The model under review builds one solid part; all positions refer to its coordinate system, in mm. A direction names the side the tool comes from. Coordinates: 2 decimals unless noted, no trailing zeros. Loops run counter-clockwise (first coordinate to the right, second up) from the corner with the lowest first, then second, coordinate; pieces in that order, holes last. Notation, with made-up numbers: M 82.5,32 L 90.5,32 A33 cw 90.5,62 Z; hole C 69.25,37 d9. An arc over 180 degrees is marked long. One line per item, written item: value.
```python
from build123d import *

# Parameters (mm, degrees)
SKETCH1_R           = 12.5
SKETCH1_R_2         = 9
BOSS_EXTRUDE1_DEPTH = 27.5
SKETCH1_3_R         = 9
BOSS_EXTRUDE2_DEPTH = 266.1
SKETCH2_R           = 12.5
BOSS_EXTRUDE3_DEPTH = 27.5


with BuildPart() as part:
    # Sketch1 → Boss-Extrude1 (new body)
    with BuildSketch(Plane(origin=(0, 0, 0), x_dir=(0, 0, -1), z_dir=(1, 0, 0))):
        Circle(SKETCH1_R)
        Circle(SKETCH1_R_2, mode=Mode.SUBTRACT)
    extrude(amount=BOSS_EXTRUDE1_DEPTH)

    # Sketch1_3 → Boss-Extrude2 (add)
    with BuildSketch(Plane(origin=(0, 0, 0), x_dir=(0, 0, -1), z_dir=(1, 0, 0))):
        Circle(SKETCH1_3_R)
    extrude(amount=BOSS_EXTRUDE2_DEPTH)

    # Sketch2 → Boss-Extrude3 (add)
    with BuildSketch(Plane(origin=(266.1, 0, 0), x_dir=(0, 0, -1), z_dir=(1, 0, 0))):
        Circle(SKETCH2_R)
    extrude(amount=-BOSS_EXTRUDE3_DEPTH)


solid = part.part
```
(1) Insertion check: pin 1 Ø3 at (x, z) = (233.5, 5.5) entering from -Y; pin 2 Ø6 at (x, z) = (65.5, 8.5) entering from -Y; pin 3 Ø3 at (x, y) = (38.5, -5.5) entering from +Z. Each pin has a flat end and moves straight along its axis. Give the tip position at first contact, or say it passes through.
Checks:
pin 1: y = -8.06
pin 2: y = -7.12
pin 3: z = 8.06
(2) Tool access review of faces 4 (the face through (238.6, 3, 9)), 5 (the face through (13.558, 3.755, -11.923)): name each direction out of +Z, -Z, +X, -X, +Y, -Y from which nothing blocks a thin tool from reaching the whole face with its end or side.
Checks:
face 4: none
face 5: +X, -X
(3) Add section C-C on x = 228. State the section outline as (y, z) points, then the cut area to 3 significant figures.
Checks:
outline: C 0,0 d18
area: 254 mm^2
(4) Draft analysis for pull direction X (two halves, no side actions). For faces 1 (the face through (252.543, 3.755, -11.923)), 2 (the face through (0, 0, 0)), 3 (the face through (27.5, 3, 9)), state which applies: pulls with the +X half, pulls with the -X half, needs draft (parallel to the pull), parting line crosses it, or undercut.
Checks:
face 1: needs draft
face 2: pulls with the -X half
face 3: undercut
(5) To check wall thickness, follow L1, parallel to X at y = 11.25, z = 2.5; L2, parallel to Y at x = 59.5, z = 0.25; L3, parallel to Y at x = 59.5, z = 6. State the ranges of each line that lie inside material, in increasing order. Write a range as [from, to].
Checks:
L1: [0, 27.5], [238.6, 266.1]
L2: [-9, 9]
L3: [-6.71, 6.71]
(6) Add section A-A on z = 0. State the section outline as (x, y) points, then the cut area to 3 significant figures.
Checks:
outline: M 0,-12.5 L 27.5,-12.5 L 27.5,-9 L 238.6,-9 L 238.6,-12.5 L 266.1,-12.5 L 266.1,12.5 L 238.6,12.5 L 238.6,9 L 27.5,9 L 27.5,12.5 L 0,12.5 Z
area: 5,170 mm^2
(7) Add section D-D on x = 17. State the section outline as (y, z) points, then the cut area to 3 significant figures.
Checks:
outline: C 0,0 d25
area: 491 mm^2
